Input: dimensioned drawing with shaded views. Units: mm. Origin: part minimum x, y, z. A direction names the side the tool comes from. Coordinates: 2 decimals unless noted, no trailing zeros. Loops run counter-clockwise (first coordinate to the right, second up) from the corner with the lowest first, then second, coordinate; pieces in that order, holes last. Notation, with made-up numbers: (32, 84) - (39, 84) arc R4 ccw to (39, 91) - close; hole circle Ø5 at (30.5, -22.75). An arc over 180 degrees is marked (long way). Use one line per item in the form item = value. Start each with the question number.
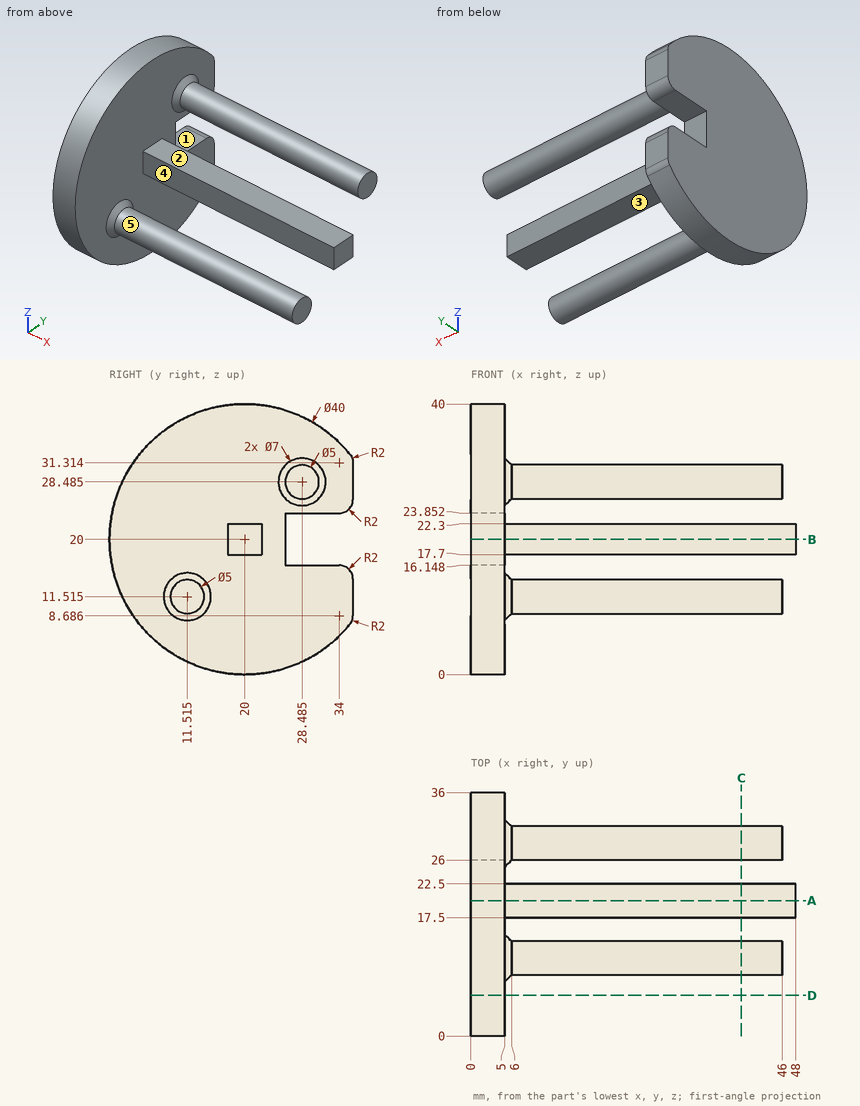
(1) Cut plane D-D, the plane y = 6. Output: boundary loops of the cut face in (x, z).
(2) Cut plane B-B, the plane z = 20. Output: boundary loops of the cut face in (x, y).
(3) Cut plane A-A, the plane y = 20. Output: boundary loops of the cut face in (x, z).
(4) Cut plane C-C, the plane x = 40. Output: boundary loops of the cut face in (y, z) (1 decimal).
(5) Access query for the marked faces 1, 2, 3, 4 and 5. Directions: +Z, -Z, +X, -X, +Y, -Y. A direction counts if a zero-diameter tool reaches every point of the face in a straight line with its end or side. Return the directions, or none.
(6) Material intervals for line 1 (X direction, y = 11.5, z = 16); line 2 (Y direction, x = 6, z = 18); line 3 (Z direction, x = 11.5, y = 21), sorted ascending.
(7) Contact query for flat-ended pins moving along their axis: pin 1 (5 mm diameter, centred on x = 5, y = 12.5, fed in from -Z) (1 decimal); pin 2 (3 mm diameter, centred on x = 7, y = 18, fed in from -Z); pin 3 (5 mm diameter, centred on x = 10, y = 10, fed in from +Z) (1 decimal). Output: stop coordinate, or through.
Recorded:
q1.outline = (0, 5.72) - (5, 5.72) - (5, 34.28) - (0, 34.28) - close
q2.outline = (0, 0) - (5, 0) - (5, 17.5) - (48, 17.5) - (48, 22.5) - (5, 22.5) - (5, 26) - (0, 26) - close
q3.outline = (0, 0) - (5, 0) - (5, 17.7) - (48, 17.7) - (48, 22.3) - (5, 22.3) - (5, 40) - (0, 40) - close
q4.outline = circle Ø5 at (11.5, 11.5); (17.5, 17.7) - (22.5, 17.7) - (22.5, 22.3) - (17.5, 22.3) - close; circle Ø5 at (28.5, 28.5)
q5.face_1 = +X, -X, +Y
q5.face_2 = +Z, +X, +Y, -Y
q5.face_3 = -Z, +X, +Y, -Y
q5.face_4 = +Z, -Z, +X, -Y
q5.face_5 = +X
q6.line_1 = 0 to 5
q6.line_2 = 17.5 to 22.5
q6.line_3 = 17.7 to 22.3
q7.pin_1 = 0.6
q7.pin_2 = 17.7
q7.pin_3 = 14
